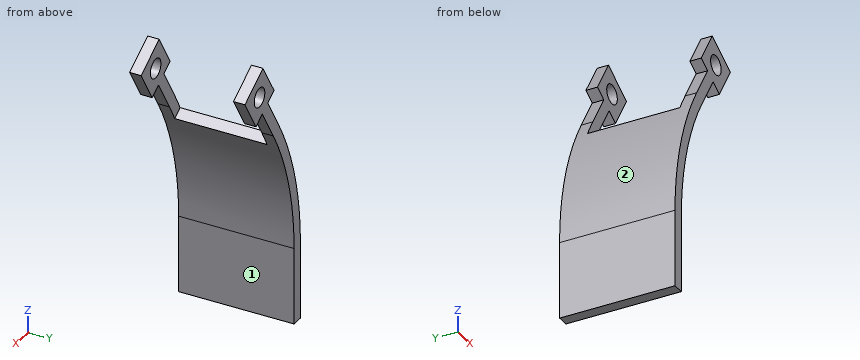
from build123d import *

# Parameters (mm, degrees)
ESQUISSE1_R      = 2.5
EXTRUSION1_DEPTH = 30
ESQUISSE3_W      = 25
ESQUISSE3_H      = 24
EXTRUSION2_DEPTH = 47.542124281


with BuildPart() as part:
    # Esquisse1 → Extrusion1 (new body)
    with BuildSketch(Plane(origin=(0, 0, 0), x_dir=(1, 0, 0), z_dir=(0, 1, 0))):
        with BuildLine():
            Line((0, 0), (0, 20))
            Line((0, 20), (3, 20))
            Line((3, 20), (3, 0))
            ThreePointArc((3, 0), (5.498625566, -18.126574307), (12.808140182, -34.901162883))
            Line((12.808140182, -34.901162883), (18.017268971, -43.437261363))
            Line((18.017268971, -43.437261363), (21.004903439, -41.614066287))
            Line((21.004903439, -41.614066287), (26.214032228, -50.150164768))
            Line((26.214032228, -50.150164768), (17.677933747, -55.359293556))
            Line((17.677933747, -55.359293556), (12.468804959, -46.823195076))
            Line((12.468804959, -46.823195076), (15.456439427, -45))
            Line((15.456439427, -45), (10.247310638, -36.46390152))
            ThreePointArc((10.247310638, -36.46390152), (2.610504323, -18.938211963), (0, 0))
        make_face()
        with Locations((19.341418593, -48.486679922)):
            Circle(ESQUISSE1_R, mode=Mode.SUBTRACT)
    extrude(amount=EXTRUSION1_DEPTH)

    # Esquisse3 → Extrusion2 (cut, through all)
    with BuildSketch(Plane(origin=(-11.734839745, 0, 7.161151161), x_dir=(0.520912879, 0, 0.853609848), z_dir=(-0.853609848, 0, 0.520912879))):
        with Locations((43.96390152, 15)):
            Rectangle(ESQUISSE3_W, ESQUISSE3_H)
    extrude(amount=-EXTRUSION2_DEPTH, mode=Mode.SUBTRACT)


solid = part.part
Geometry: final body of the model. Coordinates: model frame, mm. Face numbers are marked on the shaded views. A direction names the side the tool comes from. Round coordinates to 2 decimals unless told otherwise and drop trailing zeros. Loops run counter-clockwise (first coordinate to the right, second up) from the corner with the lowest first, then second, coordinate; pieces in that order, holes last.
Q1. Section A-A on x = 14.5. Return loops of the section in (y, z).
Q2. Section D-D on y = 28. Return loops of the section in (x, z), plus the area to 3 significant figures.
Q3. Section B-B on x = 11.5. Return loops of the section in (y, z).
Q4. Access query for the marked faces 1 and 2. Directions: +Z, -Z, +X, -X, +Y, -Y. A direction counts if a zero-diameter tool reaches every point of the face in a straight line with its end or side. Return the directions, or none.
Q5. Pin query (flat end, axial travel): P1, Ø1.5, axis at x = 8, y = 9, coming from the +Z side; P2, Ø10, axis at y = 16.5, z = -5.5, coming from the +X side. Return the tip coordinate at first contact, or that it passes through.
Q6. Material intervals for L1, parallel to Y at x = 20, z = 46; L2, parallel to X at y = 16.75, z = -7; L3, parallel to Z at x = 13.5, y = 27.75, sorted ascending.
Q7. Section C-C on z = 38.5. Return loops of the section in (x, y).
Evaluation:
1. outline: (0, 37.67) - (3, 37.67) - (3, 43.43) - (0, 43.43) - close; (0, 45.58) - (3, 45.58) - (3, 50.15) - (0, 50.15) - close; (27, 37.67) - (30, 37.67) - (30, 43.43) - (27, 43.43) - close; (27, 45.58) - (30, 45.58) - (30, 50.15) - (27, 50.15) - close
2. outline: (0, -20) - (3, -20) - (3, 0) arc R67 cw to (12.81, 34.9) - (18.02, 43.44) - (21, 41.61) - (26.21, 50.15) - (17.68, 55.36) - (12.47, 46.82) - (15.46, 45) - (10.25, 36.46) arc R70 ccw to (0, 0) - close; hole circle Ø5 at (19.34, 48.49)
2. area: 283 mm2
3. outline: (0, 32.66) - (3, 32.66) - (3, 38.52) - (0, 38.52) - close; (27, 32.66) - (30, 32.66) - (30, 38.52) - (27, 38.52) - close
4. face 1: -Z, +X, +Y, -Y
4. face 2: +Z, -X, +Y, -Y
5. P1: stops at z = 32.1
5. P2: stops at x = 3
6. L1: y = 0 to 3, 27 to 30
6. L2: x = 0 to 3
6. L3: z = 36.03 to 41.79, 46.19 to 48.51
7. outline: (11.49, 0) - (15, 0) - (15, 3) - (11.49, 3) - close; (11.49, 27) - (15, 27) - (15, 30) - (11.49, 30) - close
